from build123d import *

# Parameters (mm, degrees)
SKETCH1_R               = 35
BOSS_EXTRUDE1_DEPTH     = 10
SKETCH2_R               = 23.5
BOSS_EXTRUDE2_DEPTH     = 13
BOSS_EXTRUDE3_DEPTH     = 4
SKETCH4_R               = 1.5
CUT_EXTRUDE1_DEPTH      = 4
MIRROR2_COPY_1_SKETCH_R = 1.5
MIRROR2_COPY_1_DEPTH    = 4
BOSS_EXTRUDE4_DEPTH     = 3
SKETCH6_W               = 14
SKETCH6_H               = 26
BOSS_EXTRUDE5_DEPTH     = 2
SKETCH7_R               = 10
CUT_EXTRUDE2_DEPTH      = 10


with BuildPart() as part:
    # Sketch1 → Boss-Extrude1 (new body)
    with BuildSketch(Plane(origin=(0, 0, 0), x_dir=(0, 0, -1), z_dir=(1, 0, 0))):
        Circle(SKETCH1_R)
    extrude(amount=BOSS_EXTRUDE1_DEPTH)

    # Sketch2 → Boss-Extrude2 (add)
    with BuildSketch(Plane(origin=(10, 0, 0), x_dir=(0, 0, -1), z_dir=(1, 0, 0))):
        with Locations(Location((0, 0, 0), (0, 0, 180))):
            Circle(SKETCH2_R)
    extrude(amount=BOSS_EXTRUDE2_DEPTH)

    # Sketch3 → Boss-Extrude3 (add)
    with BuildSketch(Plane(origin=(0, 13, 0), x_dir=(1, 0, 0), z_dir=(0, 1, 0))):
        Polygon((23, 35), (23, -35), (30.392057511, -43.809511096), (35.392057511, -43.809511096), (52.433760781, -23.5), (52.433760781, 23.5), (35.392057511, 43.809511096), (30.392057511, 43.809511096), align=None)
    boss_extrude3 = extrude(amount=-BOSS_EXTRUDE3_DEPTH)

    # Sketch4 → Cut-Extrude1 (cut)
    with BuildSketch(Plane(origin=(0, 13, 0), x_dir=(1, 0, 0), z_dir=(0, 1, 0))):
        with Locations(Location((32.892057511, -40.809511096, 0), (0, 0, 270))):
            Circle(SKETCH4_R)
    cut_extrude1 = extrude(amount=-CUT_EXTRUDE1_DEPTH, mode=Mode.SUBTRACT)

    # Mirror1: Cut-Extrude1 across plane
    add(cut_extrude1.mirror(Plane.XY), mode=Mode.SUBTRACT)

    # Mirror2: Boss-Extrude3, Cut-Extrude1 across plane
    add(boss_extrude3.mirror(Plane.ZX))
    add(cut_extrude1.mirror(Plane.ZX), mode=Mode.SUBTRACT)

    # Mirror2 copy 1 sketch → Mirror2 copy 1 (cut)
    with BuildSketch(Plane.XZ.offset(13)):
        with Locations(Location((32.892057511, -40.809511096, 0), (0, 0, 270))):
            Circle(MIRROR2_COPY_1_SKETCH_R)
    extrude(amount=-MIRROR2_COPY_1_DEPTH, mode=Mode.SUBTRACT)

    # Sketch5 → Boss-Extrude4 (add)
    with BuildSketch(Plane(origin=(23, 0, 0), x_dir=(0, 0, -1), z_dir=(1, 0, 0))):
        with BuildLine():
            Line((-2, 13), (-2, 20))
            ThreePointArc((-2, 20), (0, 20.763932023), (2, 20))
            Line((2, 20), (2, 13))
            Line((2, 13), (-2, 13))
        make_face()
    boss_extrude4 = extrude(amount=BOSS_EXTRUDE4_DEPTH)

    # Mirror3: Boss-Extrude4 across plane
    add(boss_extrude4.mirror(Plane.ZX))

    # Sketch6 → Boss-Extrude5 (add)
    with BuildSketch(Plane(origin=(52.433760781, 0, 0), x_dir=(0, 0, -1), z_dir=(1, 0, 0))):
        Rectangle(SKETCH6_W, SKETCH6_H)
    extrude(amount=-BOSS_EXTRUDE5_DEPTH)

    # Sketch7 → Cut-Extrude2 (cut)
    with BuildSketch(Plane.ZY):
        Circle(SKETCH7_R)
    extrude(amount=-CUT_EXTRUDE2_DEPTH, mode=Mode.SUBTRACT)


solid = part.part
The model under review builds one solid part; all positions refer to its coordinate system, in mm. A direction names the side the tool comes from. Round coordinates to 2 decimals unless told otherwise and drop trailing zeros. Loops run counter-clockwise (first coordinate to the right, second up) from the corner with the lowest first, then second, coordinate; pieces in that order, holes last. Notation, with made-up numbers: (24.5, -38.75) -> (70.5, -38.75) arc R5 cw to (70.5, -33.75) -> close; hole circle Ø10 at (-13.75, 42.25). An arc over 180 degrees is marked (long way). One line per question, with ' | ' between items. Start each with the question number.
Item 1: Add section D-D, the plane z = 5. Write out the cut boundary in (x, y), then the cut area to 3 significant figures.
Item 2: Machinability: for faces 1 (the face through (51, 0, 7)), 2 (the face through (26, -17, 0)), 3 (the face through (24, -16, 2)), which of the approach directions +Z, -Z, +X, -X, +Y, -Y give a long, thin tool a straight path to every point of the face, cutting with its end or side? Answer none if there is none.
Item 3: Wall thickness on line 1 along Y through (x, z) = (31.5, 4.5); line 2 along X through (y, z) = (-5.5, -19); line 3 along X through (y, z) = (15, 29): over which ranges is each line inside the solid? List them lowest first. Write a range as [from, to].
Item 4: Add section B-B, the plane z = -34. Write out the cut boundary in (x, y).
Item 5: Add section A-A, the plane y = 0. Write out the cut boundary in (x, z).
Item 6: For pin 1 (1.5 mm diameter, centred on x = 25, y = 17.5, fed in from -Z); pin 2 (5 mm diameter, centred on x = 32.89, z = 40.81, fed in from +Y); pin 3 (2 mm diameter, centred on y = -16.5, z = 19, fed in from +X), all flat-tipped, find the tip position at first contact; note any pin that passes through.
Item 7: Draft analysis for pull direction Z (two halves, no side actions). For faces 4 (the face through (44.032, -11.028, -33.513)), 5 (the face through (23, 11, 27)), 6 (the face through (33, -11, 43.81)), 7 (the face through (31.43, 11.03, 40.48)), state which applies: +Z half, -Z half, draft (parallel to the pull), parting line (faces both ways), or undercut.
Item 8: Add section C-C, the plane x = 47. Write out the cut boundary in (y, z), then the cut area to 3 significant figures.
Return value:
1) outline: (0, -34.64) -> (10, -34.64) -> (10, -22.96) -> (23, -22.96) -> (23, -13) -> (52.43, -13) -> (52.43, 13) -> (23, 13) -> (23, 22.96) -> (10, 22.96) -> (10, 34.64) -> (0, 34.64) -> (0, 8.66) -> (10, 8.66) -> (10, -8.66) -> (0, -8.66) -> close; hole (23, -9) -> (50.43, -9) -> (50.43, 9) -> (23, 9) -> close | area: 1,390 mm2
2) face 1: +Z, +X | face 2: +Z, -Z, +X, -Y | face 3: +Z, +X, -Y
3) line 1: y = [-13, -9], [9, 13] | line 2: x = [0, 23] | line 3: x = [0, 10]
4) outline: (0, -8.31) -> (10, -8.31) -> (10, 8.31) -> (0, 8.31) -> close; (23, -13) -> (43.62, -13) -> (43.62, -9) -> (23, -9) -> close; (23, 9) -> (43.62, 9) -> (43.62, 13) -> (23, 13) -> close
5) outline: (0, -35) -> (10, -35) -> (10, -23.5) -> (23, -23.5) -> (23, 23.5) -> (10, 23.5) -> (10, 35) -> (0, 35) -> (0, 10) -> (10, 10) -> (10, -10) -> (0, -10) -> close; (50.43, -7) -> (52.43, -7) -> (52.43, 7) -> (50.43, 7) -> close
6) pin 1: stops at z = -2 | pin 2: stops at y = 13 | pin 3: stops at x = 10
7) face 4: -Z half | face 5: draft | face 6: +Z half | face 7: undercut
8) outline: (-13, -29.98) -> (-9, -29.98) -> (-9, 29.98) -> (-13, 29.98) -> close; (9, -29.98) -> (13, -29.98) -> (13, 29.98) -> (9, 29.98) -> close | area: 480 mm2
